Input: part model. Units: mm. Frame: model coordinates. Give positions to 0.01 mm unless a question says otherwise; leave off trailing zeros. Loops run counter-clockwise (first coordinate to the right, second up) from the corner with the lowest first, then second, coordinate; pieces in that order, holes last. Notation, with made-up numbers: M -16.5,21 L 18.5,21 A7 ccw 18.5,25 Z; hole C -24.75,-21.5 d6. An arc over 180 degrees is marked long. Return JSON: item names as keys, results as strings. Group by question number.
```python
from build123d import *

# Parameters (mm, degrees)
F1_DEPTH = 3


with BuildPart() as f1:
    # F0 (on Top) → F1 (new body)
    with BuildSketch(Plane.XY):
        Polygon((63.54102, -4.873795), (68.176275, 9.392052), (71.448817, 8.328739), (76.084072, 22.594587), (72.811529, 23.6579), (60.676275, 32.474679), (62.698817, 35.25847), (50.563562, 44.075249), (48.54102, 41.291458), (36.405765, 50.108236), (38.428307, 52.892027), (26.293052, 61.708806), (24.27051, 58.925015), (12.135255, 67.741794), (14.157797, 70.525585), (2.022542, 79.342364), (0, 76.558573), (-12.135255, 67.741794), (-14.157797, 70.525585), (-26.293052, 61.708806), (-24.27051, 58.925015), (-36.405765, 50.108236), (-38.428307, 52.892027), (-50.563562, 44.075249), (-48.54102, 41.291458), (-60.676275, 32.474679), (-62.698817, 35.25847), (-74.834072, 26.441691), (-72.811529, 23.6579), (-68.176275, 9.392052), (-71.448817, 8.328739), (-66.813562, -5.937109), (-63.54102, -4.873795), (-58.905765, -19.139643), (-62.178307, -20.202957), (-57.543052, -34.468804), (-54.27051, -33.405491), (-49.635255, -47.671339), (-52.907797, -48.734652), (-48.272542, -63.0005), (-45, -61.937186), (-30, -61.937186), (-30, -65.378141), (-15, -65.378141), (-15, -61.937186), (0, -61.937186), (0, -65.378141), (15, -65.378141), (15, -61.937186), (30, -61.937186), (30, -65.378141), (45, -65.378141), (45, -61.937186), (49.635255, -47.671339), (52.907797, -48.734652), (57.543052, -34.468804), (54.27051, -33.405491), (58.905765, -19.139643), (62.178307, -20.202957), (66.813562, -5.937109), align=None)
    extrude(amount=F1_DEPTH)


solid = f1.part
```
Item 1: Section A-A, the plane y = -51. Return loops of the section in (x, z).
Item 2: Pull-direction query (X, two-part tool) for faces 1 (the face through (66.829, 28.005, 1.479)), 2 (the face through (0, 8, 0)), 3 (the face through (-54.524, 36.945, 1.479)), 4 (the face through (-68.7, 30.9, 1.5)); classes: pulls with the +X half, pulls with the -X half, needs draft (parallel to the pull), parting line crosses it, or undercut.
Item 3: First-contact query: pin 1 Ø1.5 at (y, z) = (-63, 2) entering from -X; pin 2 Ø0.9 at (y, z) = (-64, 1.5) entering from +X; pin 3 Ø0.9 at (x, z) = (-39.5, 2) entering from -Y. Flat tips, straight axial feed; report the tip coordinate or a pass-through.
Item 4: Material intervals for line 1 (Y direction, x = 14, z = 2.85); line 2 (X direction, y = 41.5, z = 2.15); line 3 (Y direction, x = -33, z = 2.4), sorted ascending. Write a range as from..to.
Item 5: Section B-B, the plane x = -32.5. Return loops of the section in (y, z), then the cut area to 3 significant figures.
Answer below:
{
 "1": {"outline": "M -52.17,0 L 48.55,0 L 48.55,3 L -52.17,3 Z"},
 "2": {"face 1": "pulls with the +X half", "face 2": "needs draft", "face 3": "undercut", "face 4": "pulls with the -X half"},
 "3": {"pin 1": "x = -48.52", "pin 2": "x = 45", "pin 3": "y = -61.94"},
 "4": {"line 1": "-65.38..66.39, 70.31..70.64", "line 2": "-48.69..48.25, 48.69..54.11", "line 3": "-61.94..52.58"},
 "5": {"outline": "M -61.94,0 L 52.95,0 L 52.95,3 L -61.94,3 Z", "area": "345 mm^2"}
}
